Could you check a few things on this model? Use its own coordinates, in mm. Face numbers are marked on the shaded views. A direction names the side the tool comes from. Give positions to 0.01 mm unless a question says otherwise; leave off trailing zeros. Loops run counter-clockwise (first coordinate to the right, second up) from the corner with the lowest first, then second, coordinate; pieces in that order, holes last. Notation, with made-up numbers: M 9.25,63.25 L 40.25,63.25 A25 ccw 40.25,83.25 Z; hole C 85,-2.5 d5. An arc over 180 degrees is marked long. Use CSV: the item, a comma, the result in double quotes.
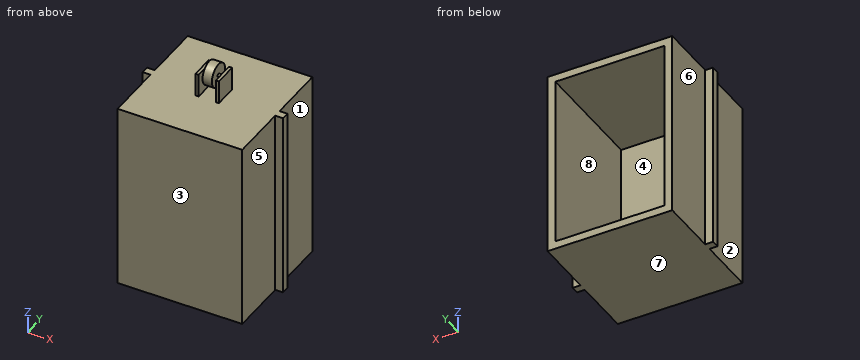
```python
from build123d import *

# Parameters (mm, degrees)
SKETCH1_W                = 400
SKETCH1_H                = 400
BOSS_EXTRUDE1_DEPTH      = 600
SKETCH2_W                = 350
SKETCH2_H                = 550
CUT_EXTRUDE1_DEPTH       = 375
SKETCH3_W                = 25
SKETCH3_H                = 25
BOSS_EXTRUDE2_DEPTH      = 600
SKETCH4_W                = 75
SKETCH4_H                = 75
BOSS_EXTRUDE3_DEPTH      = 75
SKETCH5_W                = 55
SKETCH5_H                = 75
CUT_EXTRUDE2_DEPTH       = 75
BOSS_EXTRUDE4_START      = -22.5
SKETCH6_R                = 37.5
BOSS_EXTRUDE4_DEPTH      = 30
BOSS_EXTRUDE5_DEPTH      = 22
BOSS_EXTRUDE5_DEPTH_BACK = 44
SKETCH7_R                = 5


with BuildPart() as part:
    # Sketch1 → Boss-Extrude1 (new body)
    with BuildSketch(Plane.XY):
        with Locations((200, -200)):
            Rectangle(SKETCH1_W, SKETCH1_H)
    extrude(amount=BOSS_EXTRUDE1_DEPTH)

    # Sketch2 → Cut-Extrude1 (cut)
    with BuildSketch(Plane(origin=(0, 0, 0), x_dir=(1, 0, 0), z_dir=(0, 1, 0))):
        with Locations((200, -300)):
            Rectangle(SKETCH2_W, SKETCH2_H)
    extrude(amount=-CUT_EXTRUDE1_DEPTH, mode=Mode.SUBTRACT)

    # Sketch3 → Boss-Extrude2 (add)
    with BuildSketch(Plane.XY.offset(600)):
        with Locations((412.5, -200)):
            Rectangle(SKETCH3_W, SKETCH3_H)
        with Locations((-12.5, -200)):
            Rectangle(SKETCH3_W, SKETCH3_H)
    extrude(amount=-BOSS_EXTRUDE2_DEPTH)

    # Sketch4 → Boss-Extrude3 (add)
    with BuildSketch(Plane.XY.offset(600)):
        with Locations((196.145511261, -200)):
            Rectangle(SKETCH4_W, SKETCH4_H)
    extrude(amount=BOSS_EXTRUDE3_DEPTH)

    # Sketch5 → Cut-Extrude2 (cut)
    with BuildSketch(Plane(origin=(0, -162.5, 0), x_dir=(1, 0, 0), z_dir=(0, 1, 0))):
        with Locations((196.145511261, -637.5)):
            Rectangle(SKETCH5_W, SKETCH5_H)
    extrude(amount=-CUT_EXTRUDE2_DEPTH, mode=Mode.SUBTRACT)



with BuildPart() as body_2:
    # Sketch6 → Boss-Extrude4 (new body)
    with BuildSketch(Plane(origin=(233.645511261, 0, 0), x_dir=(0, 0, -1), z_dir=(1, 0, 0)).offset(BOSS_EXTRUDE4_START)):
        with Locations((-665, -200)):
            Circle(SKETCH6_R)
    extrude(amount=-BOSS_EXTRUDE4_DEPTH)


with BuildPart() as part_1:
    add(part.part)

    add(body_2.part)  # Boss-Extrude5 merges body 2
    # Sketch7 → Boss-Extrude5 (add, two sides: drawn at the far end of the back side and taken through both)
    with BuildSketch(Plane(origin=(211.145511261, 0, 0), x_dir=(0, 0, -1), z_dir=(1, 0, 0)).offset(-BOSS_EXTRUDE5_DEPTH_BACK)):
        with Locations((-665, -200)):
            Circle(SKETCH7_R)
    extrude(amount=BOSS_EXTRUDE5_DEPTH + BOSS_EXTRUDE5_DEPTH_BACK)


solid = part_1.part
```
1. I want a section at D-D, the plane z = 640.5. List the corners of the cut face in (x, y) for me.
Outcome:
outline,"M 158.65,-237.5 L 168.65,-237.5 L 168.65,-162.5 L 158.65,-162.5 Z; M 181.15,-228.39 L 211.15,-228.39 L 211.15,-171.61 L 181.15,-171.61 Z; M 223.65,-237.5 L 233.65,-237.5 L 233.65,-162.5 L 223.65,-162.5 Z"
2. If we mould it in two halves opening along X, with no side actions, what happens to the marked faces 5, 6, 7 and 8? For each: +X half, -X half, draft (parallel to the pull), parting line (faces both ways), or undercut.
Outcome:
face 5,"+X half"
face 6,"-X half"
face 7,"draft"
face 8,"undercut"
3. Please list where these lines run through material, in increasing order: line 1 (X direction, y = -105, z = 163.5); line 2 (Z direction, x = 74, y = -369); line 3 (Y direction, x = 123.5, z = 327.5).
Outcome:
line 1,"0 to 25, 375 to 400"
line 2,"0 to 25, 575 to 600"
line 3,"-400 to -375"
4. I'm going to push flat-ended pins straight in: pin 1 Ø3 at (y, z) = (-217, 549) entering from +X; pin 2 Ø11 at (x, z) = (164.5, 634) entering from -Y; pin 3 Ø8 at (x, y) = (229, -137) entering from +Z. Where does each tip first touch, or does it pass through?
Outcome:
pin 1,"x = 400"
pin 2,"y = -237.5"
pin 3,"z = 600"
5. I want a section at C-C, the plane x = 79.5. List the corners of the cut face in (y, z) for me, then the cut area to 4 significant figures.
Outcome:
outline,"M -400,0 L 0,0 L 0,25 L -375,25 L -375,575 L 0,575 L 0,600 L -400,600 Z"
area,"33,750 mm2"
6. I want a section at A-A, the plane y = -67. List the corners of the cut face in (x, z) for me, then the cut area to 3 significant figures.
Outcome:
outline,"M 0,0 L 400,0 L 400,600 L 0,600 Z; hole M 25,25 L 375,25 L 375,575 L 25,575 Z"
area,"47,500 mm2"
7. I want a section at B-B, the plane y = -224.5. List the corners of the cut face in (x, z) for me.
Outcome:
outline,"M 0,0 L 400,0 L 400,600 L 233.65,600 L 233.65,675 L 223.65,675 L 223.65,600 L 168.65,600 L 168.65,675 L 158.65,675 L 158.65,600 L 0,600 Z; M 181.15,636.61 L 211.15,636.61 L 211.15,693.39 L 181.15,693.39 Z; hole M 25,25 L 375,25 L 375,575 L 25,575 Z"
8. Which directions (+Z, -Z, +X, -X, +Y, -Y) give clear straight access to the entire face, cutting with the end or side of a thin tool? Please do the marked faces 1, 2, 3 and 4.
Outcome:
face 1,"+Z, -Z, +X, +Y"
face 2,"+Z, -Z, -X, -Y"
face 3,"+Z, -Z, +X, -X, -Y"
face 4,"+Y"
